The model under review builds one solid part; all positions refer to its coordinate system, in mm. A direction names the side the tool comes from. Round coordinates to 2 decimals unless told otherwise and drop trailing zeros. Loops run counter-clockwise (first coordinate to the right, second up) from the corner with the lowest first, then second, coordinate; pieces in that order, holes last. Notation, with made-up numbers: (-10, 27.5) -> (-6, 27.5) arc R15 ccw to (-6, 49.5) -> close; hole circle Ø10 at (-3, -30.75). An arc over 180 degrees is marked (long way). Write each question's results on one line, items separated by ' | '. Start each with the question number.
Item 1: For L1, parallel to X at y = -76.5, z = -4.5; L2, parallel to Z at x = 7.25, y = -62; L3, parallel to X at y = -8, z = 28.5, list the stretches that pass through material, from the lowest coordinate up. Write a range as from..to.
Item 2: Clearance check with flat-ended pins moving along their axes: pin 1 Ø2 at (y, z) = (-107.5, -6) entering from +X; pin 2 Ø5 at (y, z) = (-66, 30.5) entering from +X; pin 3 Ø3 at (y, z) = (-133.5, 10) entering from +X. State where each tip first meets the part, or that it passes through.
Item 3: We need section A-A (x = -1.5). Give the boundary of the cut face in (y, z).
Item 4: Tool access review of faces 1 (the flat face through (-6, -75, 38.071)), 2 (the flat face through (3.168, -75, 29)): name each direction out of +Z, -Z, +X, -X, +Y, -Y from which nothing blocks a thin tool from reaching the whole face with its end or side.
from build123d import *

# Parameters (mm, degrees)
F1_DEPTH = 152.4


# Not quite as in the source:
# - ends of sketch curves that miss each other by under 0.0002 mm in the source are joined
# - the dataset's text gives a spline's control points without its knots; the knots are read off the source's solid


with BuildPart() as f1:
    # F0 (on Front) → F1 (new body)
    with BuildSketch(Plane.XZ):
        with BuildLine():
            Line((9.5127572, -38.0712472), (9.5127572, 7.931531))
            add(Edge.make_bspline(
                [(6.3401448, 15.1268176), (5.8891424, 14.1770608), (4.9154588, 12.1265696), (6.532499, 8.7763096), (8.6041992, 8.1890616), (9.5127572, 7.931531)],
                knots=[0, 0, 0, 0, 0.120135, 0.259368, 0.368128, 0.368128, 0.368128, 0.368128], degree=3))
            add(Edge.make_bspline(
                [(3.1675578, 26.9671546), (4.9711102, 26.507059), (8.7999316, 25.5303274), (10.3429562, 18.8598302), (7.5847956, 16.2875722), (6.3401448, 15.1268176)],
                knots=[0, 0, 0, 0, 0.207787, 0.441117, 0.632993, 0.632993, 0.632993, 0.632993], degree=3))
            Line((3.1675578, 26.9671546), (3.1675578, 31.7260478))
            ThreePointArc((3.1675578, 31.7260478), (-1.3191757237, 33.5845390763), (-3.1776416, 38.0712726))
            Line((-3.1776416, 38.0712726), (-9.5228664, 38.0712726))
            Line((-9.5228664, 38.0712726), (-9.5228664, -38.0712472))
            Line((-9.5228664, -38.0712472), (9.5127572, -38.0712472))
        make_face()
    extrude(amount=F1_DEPTH)


solid = f1.part
Here are the results:
1) L1: x = -9.52..9.51 | L2: z = -38.07..8.83, 15.99..25.4 | L3: x = -9.52..3.17
2) pin 1: stops at x = 9.51 | pin 2: stops at x = 3.17 | pin 3: stops at x = 7.84
3) outline: (-152.4, -38.07) -> (0, -38.07) -> (0, 33.77) -> (-152.4, 33.77) -> close
4) face 1: +Z, +X, -X, +Y, -Y | face 2: +Z, +X, +Y, -Y
